Could you check a few things on this model? Use its own coordinates, in mm. A direction names the side the tool comes from. Give positions to 0.01 mm unless a question says otherwise; leave off trailing zeros. Write each loop counter-clockwise with the first axis right and the second up, starting at its lowest first coordinate (ties: lowest second). Pieces come first, ordered by that corner, then holes. Notation, with made-up numbers: (-17.75, -26.75) -> (24.25, -26.75) arc R29 ccw to (24.25, 5.25) -> close; hole circle Ø9 at (18, 73.25). An arc over 180 degrees is marked (long way). One line per question, with ' | ' between items.
Autodesk Inventor part; units mm, degrees
ref_plane "YZ Plane" through (0, 0, 0) normal (1, 0, 0) x (0, 1, 0)
ref_plane "XZ Plane" through (0, 0, 0) normal (0, 1, 0) x (-1, 0, 0)
ref_plane "XY Plane" through (0, 0, 0) normal (0, 0, 1) x (1, 0, 0)
sketch "Эскиз1" plane through (0, 0, 0) normal (0, 0, 1) x (1, 0, 0)
  line L0 (-45, -15) -> (45, -15)
  line L1 (45, 15) -> (-45, 15)
  line L2 (-45, 15) -> (-45, -15)
  line L3 (-45, -15) -> (45, 15) construction
  line L4 (45, -15) -> (-45, 15) construction
  line L5 (45, 14) -> (37, 6)
  line L6 (37, 6) -> (34, 6)
  line L7 (34, 6) -> (34, 0)
  line L8 (34, 0) -> (45, 0) construction
  line L9 (45, -14) -> (37, -6)
  line L10 (37, -6) -> (34, -6)
  line L11 (34, -6) -> (34, 0)
  line L12 (-13, 0) -> (9, 0) construction
  line L13 (-13, -4) -> (9, -4)
  line L14 (9, 4) -> (-13, 4)
  arc A0 (-13, 4) -> (-13, -4) centre (-13, 0) ccw
  arc A1 (9, -4) -> (9, 4) centre (9, 0) ccw
  line L15 (45, -15) -> (45, -14)
  line L16 (45, 14) -> (45, 15)
  circle A2 centre (51.5061, 0) radius 14.5 construction
  point P0 (0, 0)
  point P1 (0, 0)
  point P2 (-2, 0)
  point P3 (0, 0)
  dimension "d0" = 90
  dimension "d1" = 28
  dimension "d2" = 12
  dimension "d3" = 30
  dimension "d4" = 90
  dimension "d5" = 4
  dimension "d6" = 22
  dimension "d7" = 36
  dimension "d9" = 11
  dimension "d17" = 29
  dimension "d18" = 6.5061
extrude "Выдавливание1" add sketch "Эскиз1" against normal blind 36 contours L2 L1 L16 L5 L6 L7 L11 L10 L9 L15 L0 | A0 L14 A1 L13
extrude "Выдавливание2" cut sketch "Эскиз1" against normal blind 2 contours A0 L14 A1 L13
mirror "Зеркальное отражение1" about plane through (1.1429, 0, -36) normal (0, 0, -1)
chamfer "Фаска1" distance 2 angle 45 2 edges at (-45, 15, -36) (-45, -15, -36)
properties part number "Призма 5"
Q1. Imagine slicing it at A-A on y = 0. Please give me the cut outline in (x, z), and give its area (3 significant figures).
Answer below:
outline: (-45, -72) -> (-17, -72) -> (-17, -70) -> (13, -70) -> (13, -72) -> (34, -72) -> (34, 0) -> (13, 0) -> (13, -2) -> (-17, -2) -> (-17, 0) -> (-45, 0) -> close | area: 5,570 mm^2
Q2. Imagine slicing it at C-C on y = 10.5. Please give me the cut outline in (x, z), and give its area (3 significant figures).
Answer below:
outline: (-45, -72) -> (41.5, -72) -> (41.5, 0) -> (-45, 0) -> close | area: 6,230 mm^2
Q3. If I drill on line 1 along X through (y, z) = (-0.5, -67.5); line 2 along Y through (x, z) = (36.5, -8.5); line 3 along Z through (x, y) = (9, 3.5), over which ranges is the centre line in solid material (lowest first)?
Answer below:
line 1: x = -45 to 34 | line 2: y = -15 to -6, 6 to 15 | line 3: z = -70 to -2
Q4. If we mould it in two halves opening along X, with no side actions, what happens to faces 6 (the flat face through (36, -6, -35)), 7 (the cylindrical face through (-17, 0, -1)), 8 (the flat face through (41, -10, -35)), 9 (the flat face through (-44, 14, -37))? For each: +X half, -X half, draft (parallel to the pull), parting line (faces both ways), or undercut.
Answer below:
face 6: draft | face 7: undercut | face 8: +X half | face 9: -X half
Q5. Imagine slicing it at B-B on z = -8. Please give me the cut outline in (x, y).
Answer below:
outline: (-45, -13) -> (-43, -15) -> (45, -15) -> (45, -14) -> (37, -6) -> (34, -6) -> (34, 6) -> (37, 6) -> (45, 14) -> (45, 15) -> (-43, 15) -> (-45, 13) -> close
Q6. On a 3-axis mill with a long thin cutter (end or side, diameter ignored), from which of +Z, -Z, +X, -X, +Y, -Y can I reach the whole of each face in a straight line? I mean faces 1 (the flat face through (-44, -14, -35)), 2 (the flat face through (2, 15, -35)), 3 (the flat face through (36, 6, -35)), 4 (the cylindrical face through (13, 0, -1)), 5 (the flat face through (-2, -4, -71)). Say none if no direction works.
Answer below:
face 1: +Z, -Z, -X, -Y | face 2: +Z, -Z, +X, -X, +Y | face 3: +Z, -Z, +X | face 4: +Z | face 5: -Z
Q7. Will these pins go through, and if not, where does the flat tip stop? pin 1 (2.5 mm diameter, centred on x = 5, y = -0.5, fed in from +Z); pin 2 (5 mm diameter, centred on x = 24.5, y = -4, fed in from +Z); pin 3 (13 mm diameter, centred on y = 1, z = -21.5, fed in from +X).
Answer below:
pin 1: stops at z = -2 | pin 2: stops at z = 0 | pin 3: stops at x = 38.5
